from build123d import *

# Parameters (mm, degrees)
F0_R     = 8.3591394984
F0_R_2   = 8.7902247906
F1_DEPTH = 6


# Not quite as in the source:
# - a feature names something its author has since deleted; it is built from what else it names


with BuildPart() as f1:
    # F0 (on Front) → F1 (new body)
    with BuildSketch(Plane.XZ):
        with BuildLine():
            Line((100.5853836174, -74.9584571321), (110.5853836174, -74.9584571321))
            add(Edge.make_bspline(
                [(110.5853836174, -74.9584571321), (126.6854561112, -57.248377389), (128.3848433658, 59.317552439), (128.5642162874, 85.0415428679)],
                knots=[0, 0, 0, 0, 148.4595862799, 148.4595862799, 148.4595862799, 148.4595862799], degree=3))
            Line((128.5642162874, 85.0415428679), (109.5853836174, 85.0415428679))
            Line((109.5853836174, 85.0415428679), (90.5853836174, 85.0415428679))
            Line((90.5853836174, 85.0415428679), (90.5853836174, -54.9584571321))
            Line((90.5853836174, -54.9584571321), (100.5853836174, -54.9584571321))
            Line((100.5853836174, -54.9584571321), (100.5853836174, -74.9584571321))
        make_face()
        with Locations((109.0683937073, 19.6757875151)):
            Circle(F0_R, mode=Mode.SUBTRACT)
        with Locations((108.2727760077, 66.6170529789)):
            Circle(F0_R_2, mode=Mode.SUBTRACT)
        with BuildLine():
            add(Edge.make_bspline(
                [(128.5642162874, 85.0415428679), (128.5853836174, 88.0771637948), (128.5853836174, 89.8477431573), (128.5853836174, 90.0415428679)],
                knots=[148.4595862799, 148.4595862799, 148.4595862799, 148.4595862799, 165.9789143235, 165.9789143235, 165.9789143235, 165.9789143235], degree=3))
            Line((128.5853836174, 90.0415428679), (109.5853836174, 90.0415428679))
            Line((109.5853836174, 90.0415428679), (109.5853836174, 85.0415428679))
            Line((109.5853836174, 85.0415428679), (128.5642162874, 85.0415428679))
        make_face()
        with BuildLine():
            Line((109.5853836174, 90.0415428679), (128.5853836174, 90.0415428679))
            add(Edge.make_bspline(
                [(128.5642162874, 95.0415428679), (128.5853836174, 92.005921941), (128.5853836174, 90.2353425785), (128.5853836174, 90.0415428679)],
                knots=[148.4595862799, 148.4595862799, 148.4595862799, 148.4595862799, 165.9789143235, 165.9789143235, 165.9789143235, 165.9789143235], degree=3))
            Line((128.5642162874, 95.0415428679), (109.5853836174, 95.0415428679))
            Line((109.5853836174, 95.0415428679), (109.5853836174, 90.0415428679))
        make_face()
        with BuildLine():
            Line((109.5853836174, 95.0415428679), (128.5642162874, 95.0415428679))
            add(Edge.make_bspline(
                [(110.5853836174, 255.0415428679), (126.6854561112, 237.3314631248), (128.3848433658, 120.7655332968), (128.5642162874, 95.0415428679)],
                knots=[0, 0, 0, 0, 148.4595862799, 148.4595862799, 148.4595862799, 148.4595862799], degree=3))
            Line((110.5853836174, 255.0415428679), (100.5853836174, 255.0415428679))
            Line((100.5853836174, 255.0415428679), (100.5853836174, 235.0415428679))
            Line((100.5853836174, 235.0415428679), (90.5853836174, 235.0415428679))
            Line((90.5853836174, 235.0415428679), (90.5853836174, 95.0415428679))
            Line((90.5853836174, 95.0415428679), (109.5853836174, 95.0415428679))
        make_face()
        with Locations((108.2727760077, 113.4660327569)):
            Circle(F0_R_2, mode=Mode.SUBTRACT)
        with Locations((109.0683937073, 160.4072982207)):
            Circle(F0_R, mode=Mode.SUBTRACT)
    extrude(amount=F1_DEPTH)


solid = f1.part
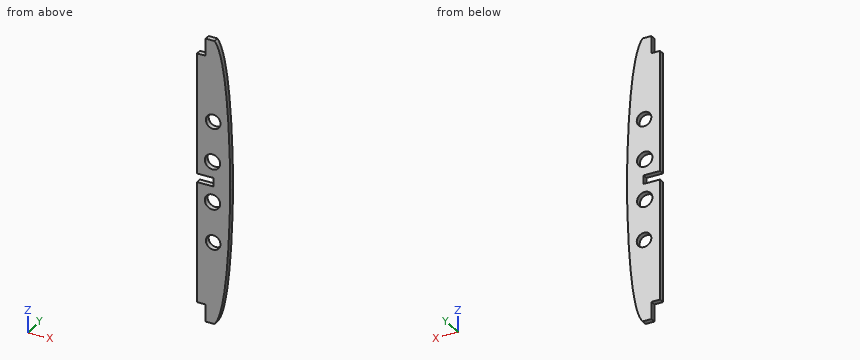
Source: CAD feature listing. Evaluate the final solid. Frame: model axes, mm. Coordinates: 2 decimals unless noted, no trailing zeros. Write each loop counter-clockwise with the first axis right and the second up, starting at its lowest first coordinate (ties: lowest second). Pieces come first, ordered by that corner, then holes. Notation, with made-up numbers: M 31,-18.75 L 69,-18.75 A21 ccw 69,0.25 Z; hole C 69,79.5 d8. An arc over 180 degrees is marked long. Use a Markdown table: item, result.
1) First-contact query: pin 1 Ø3 at (x, y) = (96.5, -2) entering from +Z; pin 2 Ø14 at (x, z) = (108.27, 66.62) entering from +Y (1 decimal); pin 3 Ø1.8 at (x, y) = (95, -3.5) entering from -Z; pin 4 Ø1.8 at (y, z) = (-4, -62.5) entering from -X. Flat tips, straight axial feed; report the tip coordinate or a pass-through.
Conclusion:
| item | result |
|---|---|
| pin 1 | stops at z = 235.04 |
| pin 2 | passes through |
| pin 3 | stops at z = -54.96 |
| pin 4 | stops at x = 100.59 |
2) Ray query, L1, parallel to Z at x = 108.5, y = -5.25; L2, parallel to Z at x = 97, y = -3.25; L3, parallel to Z at x = 107.5, y = -2.75. Return the intervals inside material, ascending.
Conclusion:
| item | result |
|---|---|
| L1 | z = -74.96 to 11.34, 28.02 to 57.83, 75.4 to 85.04, 95.04 to 104.68, 122.25 to 152.07, 168.75 to 255.04 |
| L2 | z = -54.96 to 85.04, 95.04 to 235.04 |
| L3 | z = -74.96 to 11.47, 27.89 to 57.86, 75.37 to 85.04, 95.04 to 104.71, 122.22 to 152.2, 168.62 to 255.04 |
3) Section B-B, the plane y = -4. Give the number of separate pieces and of enclosed holes in the cut face, then the cut area to 3 significant figures.
Conclusion:
| item | result |
|---|---|
| separate pieces | 1 |
| enclosed holes | 4 |
| area | 9,630 mm^2 |
4) Section A-A, the plane x = 95.5. Output: boundary loops of the cut face in (y, z).
Conclusion:
| item | result |
|---|---|
| outline | M -6,-54.96 L 0,-54.96 L 0,85.04 L -6,85.04 Z; M -6,95.04 L 0,95.04 L 0,235.04 L -6,235.04 Z |
